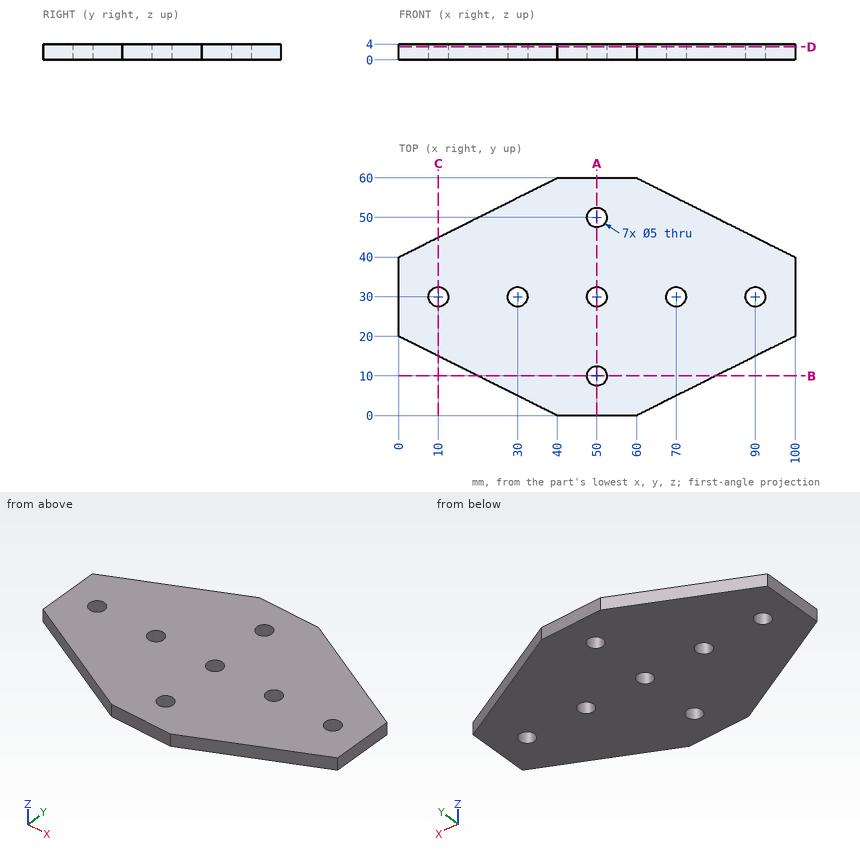
The drawing under review shows one solid part. Ordinate dimensions are in mm from its lowest x, y, z. Coordinates: 2 decimals unless noted, no trailing zeros. Order: outer loops, then holes, each group sorted by start corner. A loop starts at its lowest first (then second) coordinate and runs counter-clockwise, first axis right, second up. Notation, with made-up numbers: M -28,7.25 L 6,7.25 A32 ccw 6,40.25 Z; hole C -18.5,61.25 d10. An arc over 180 degrees is marked long. One line per question, with ' | ' between items.
(1) Add section B-B, the plane y = 10. Write out the cut boundary in (x, z), then the cut area to 3 significant figures.
Geometry results:
outline: M 20,0 L 47.5,0 L 47.5,4 L 20,4 Z; M 52.5,0 L 80,0 L 80,4 L 52.5,4 Z | area: 220 mm²
(2) Insertion check: pin 1 (2 mm diameter, centred on x = 69.5, z = 3, fed in from -Y); pin 2 (4.5 mm diameter, centred on x = 50, y = 10, fed in from +Z). Each pin has a flat end and moves straight along its axis. Give the tip position at first contact, or say it passes through.
Geometry results:
pin 1: stops at y = 4.25 | pin 2: passes through
(3) Add section C-C, the plane x = 10. Write out the cut boundary in (y, z), then the cut area to 4 significant figures.
Geometry results:
outline: M 15,0 L 27.5,0 L 27.5,4 L 15,4 Z; M 32.5,0 L 45,0 L 45,4 L 32.5,4 Z | area: 100.0 mm²
(4) For probe 1 along X at (y, z) = (30, 0.9); probe 2 along Y at (x, z) = (50, 2.7); probe 3 along X at (y, z) = (31, 2.85), list the stretches that pass through material, from the lowest coordinate up. Write a range as from..to.
Geometry results:
probe 1: x = 0..7.5, 12.5..27.5, 32.5..47.5, 52.5..67.5, 72.5..87.5, 92.5..100 | probe 2: y = 0..7.5, 12.5..27.5, 32.5..47.5, 52.5..60 | probe 3: x = 0..7.71, 12.29..27.71, 32.29..47.71, 52.29..67.71, 72.29..87.71, 92.29..100
(5) Add section A-A, the plane x = 50. Write out the cut boundary in (y, z), then the cut area to 3 significant figures.
Geometry results:
outline: M 0,0 L 7.5,0 L 7.5,4 L 0,4 Z; M 12.5,0 L 27.5,0 L 27.5,4 L 12.5,4 Z; M 32.5,0 L 47.5,0 L 47.5,4 L 32.5,4 Z; M 52.5,0 L 60,0 L 60,4 L 52.5,4 Z | area: 180 mm²
(6) Add section D-D, the plane z = 3.25. Write out the cut boundary in (x, y).
Geometry results:
outline: M 0,20 L 40,0 L 60,0 L 100,20 L 100,40 L 60,60 L 40,60 L 0,40 Z; hole C 10,30 d5; hole C 30,30 d5; hole C 50,10 d5; hole C 50,30 d5; hole C 50,50 d5; hole C 70,30 d5; hole C 90,30 d5
